The listing builds one solid part. Answer for the finished solid, in the listing's coordinates (mm). Face numbers are marked on the shaded views. A direction names the side the tool comes from. Give positions to 0.01 mm unless a question says otherwise; leave off trailing zeros. Write each loop counter-clockwise with the first axis right and the second up, starting at its lowest first coordinate (ties: lowest second). Pieces come first, ordered by that corner, then holes. Notation, with made-up numbers: M 53.5,52 L 94.5,52 A15 cw 94.5,71 Z; hole C 16,74.25 d3. An arc over 180 degrees is marked long. Answer as a JSON object with one key per item and string values.
Autodesk Inventor part; units mm, degrees
ref_plane "YZ Plane" through (0, 0, 0) normal (1, 0, 0) x (0, 1, 0)
ref_plane "XZ Plane" through (0, 0, 0) normal (0, 1, 0) x (-1, 0, 0)
ref_plane "XY Plane" through (0, 0, 0) normal (0, 0, 1) x (1, 0, 0)
sketch "Esquisse1" plane through (0, 0, 0) normal (0, 1, 0) x (-1, 0, 0)
  line L0 (0, 5) -> (40, 5)
  line L1 (40, 5) -> (40, -5)
  line L2 (40, -5) -> (0, -5)
  line L3 (0, -5) -> (0, 5)
  line L4 (0, 5) -> (17.5, 5)
  line L5 (17.5, 5) -> (17.5, 19)
  line L6 (17.5, 19) -> (0, 19)
  line L7 (0, 19) -> (0, 5)
  line L8 (0, -5) -> (12.7, -5)
  line L9 (12.7, -5) -> (12.7, -12.2)
  line L10 (12.7, -12.2) -> (0, -12.2)
  line L11 (0, -12.2) -> (0, -5)
  line L12 (17.5, 5) -> (21.5, 5)
  line L13 (21.5, 5) -> (21.5, 7)
  line L14 (21.5, 7) -> (17.5, 7)
  line L15 (17.5, 7) -> (17.5, 5)
  line L16 (12.7, -5) -> (14.7, -5)
  line L17 (14.7, -5) -> (14.7, -7)
  line L18 (14.7, -7) -> (12.7, -7)
  line L19 (12.7, -7) -> (12.7, -5)
  line L20 (40, -5) -> (14.7, -5)
  line L21 (14.7, -5) -> (14.7, -7)
  line L22 (14.7, -7) -> (40, -7)
  line L23 (40, -7) -> (40, -5)
  line L24 (12.7, -12.2) -> (14.7, -12.2)
  line L25 (14.7, -12.2) -> (14.7, -7)
  line L26 (14.7, -7) -> (12.7, -7)
  line L27 (12.7, -7) -> (12.7, -12.2)
  line L28 (40, 5) -> (21.5, 5)
  line L29 (21.5, 5) -> (21.5, 7)
  line L30 (21.5, 7) -> (40, 7)
  line L31 (40, 7) -> (40, 5)
  line L32 (21.5, 7) -> (17.5, 7)
  line L33 (17.5, 7) -> (17.5, 19)
  line L34 (17.5, 19) -> (21.5, 19)
  line L35 (21.5, 19) -> (21.5, 7)
  line L36 (40, -5) -> (42, -5)
  line L37 (42, -5) -> (42, 5)
  line L38 (42, 5) -> (40, 5)
  line L39 (40, 5) -> (40, -5)
  line L40 (0, -12.2) -> (12.7, -12.2)
  line L41 (12.7, -12.2) -> (12.7, -12.7)
  line L42 (12.7, -12.7) -> (0, -12.7)
  line L43 (0, -12.7) -> (0, -12.2)
  line L44 (0, 19) -> (17.5, 19)
  line L45 (17.5, 19) -> (17.5, 19.5)
  line L46 (17.5, 19.5) -> (0, 19.5)
  line L47 (0, 19.5) -> (0, 19)
  line L48 (21.5, 19) -> (17.5, 19)
  line L49 (17.5, 19) -> (17.5, 19.5)
  line L50 (17.5, 19.5) -> (21.5, 19.5)
  line L51 (21.5, 19.5) -> (21.5, 19)
  line L52 (42, 5) -> (40, 5)
  line L53 (40, 5) -> (40, 7)
  line L54 (40, 7) -> (42, 7)
  line L55 (42, 7) -> (42, 5)
  line L56 (42, -5) -> (40, -5)
  line L57 (40, -5) -> (40, -7)
  line L58 (40, -7) -> (42, -7)
  line L59 (42, -7) -> (42, -5)
  line L60 (14.7, -12.2) -> (12.7, -12.2)
  line L61 (12.7, -12.2) -> (12.7, -12.7)
  line L62 (12.7, -12.7) -> (14.7, -12.7)
  line L63 (14.7, -12.7) -> (14.7, -12.2)
  line L64 (0, 19.5) -> (21.5, 19.5)
  line L65 (21.5, 19.5) -> (21.5, 25.5)
  line L66 (21.5, 25.5) -> (0, 25.5)
  line L67 (0, 25.5) -> (0, 19.5)
  line L68 (0, -12.7) -> (14.7, -12.7)
  line L69 (14.7, -12.7) -> (14.7, -18.7)
  line L70 (14.7, -18.7) -> (0, -18.7)
  line L71 (0, -18.7) -> (0, -12.7)
  line L72 (42, -7) -> (56, -7)
  line L73 (56, -7) -> (56, 7)
  line L74 (56, 7) -> (42, 7)
  line L75 (42, 7) -> (42, -7)
  arc A0 (56, 7) -> (21.5, 25.5) centre (10.75, -35.9662) ccw
  arc A1 (21.5, 25.5) -> (0, 25.5) centre (10.75, -35.9662) ccw construction
  arc A2 (0, -18.7) -> (14.7, -18.7) centre (7.35, 85.9876) ccw construction
  arc A3 (14.7, -18.7) -> (56, -7) centre (7.35, 85.9876) ccw
  point P0 (0, 0)
  point P1 (0, 0)
  dimension "d1" = 40
  dimension "d3" = 14
  dimension "d4" = 10
  dimension "d5" = 7.2
  dimension "d6" = 0.5
  dimension "d7" = 0.5
  dimension "d8" = 17.5
  dimension "d9" = 12.7
  dimension "d10" = 2
  dimension "d11" = 2
  dimension "d12" = 2
  dimension "d13" = 4
  dimension "d14" = 2
  dimension "d15" = 6
  dimension "d16" = 6
  dimension "d17" = 14
extrude "Extrusion1" add sketch "Esquisse1" along normal mid plane 26 contours L67 L66 L65 L50 L46 | L35 L51 L65 A0 L74 L54 L30 | L42 L62 L69 L70 L71 | L55 L74 L73 L72 L59 L37 | L22 L58 L72 A3 L69 L63 L25
mirror "Symétrie1" about plane through (0, 0, 0) normal (1, 0, 0) of "Extrusion1"
sketch "Esquisse4" plane through (-14.7, -13, -18.7) normal (0, 0, -1) x (-1, 0, 0)
  circle A0 centre (-14.7, 13) radius 9.5
  dimension "d25" = 19
extrude "Extrusion4" cut sketch "Esquisse4" against normal through all
sketch "Esquisse5" plane through (0, 13, 0) normal (0, 1, 0) x (1, 0, 0)
  circle A0 centre (19.7, 12) radius 3.5
  circle A1 centre (28.5, -14) radius 3.5
  line L0 (42, 7) -> (56, -7) construction
  line L1 (56, 7) -> (42, -7) construction
  circle A2 centre (49, 0) radius 3.5
  line L2 (21.5, -7) -> (35.5, -7) construction
  line L3 (35.5, -7) -> (35.5, -21) construction
  line L4 (35.5, -21) -> (21.5, -21) construction
  line L5 (21.5, -21) -> (21.5, -7) construction
  line L6 (14.7, 7) -> (24.7, 7) construction
  line L7 (24.7, 7) -> (24.7, 17) construction
  line L8 (24.7, 17) -> (14.7, 17) construction
  line L9 (14.7, 17) -> (14.7, 7) construction
  line L10 (14.7, 17) -> (24.7, 7) construction
  line L11 (24.7, 17) -> (14.7, 7) construction
  line L12 (21.5, -7) -> (35.5, -21) construction
  line L13 (35.5, -7) -> (21.5, -21) construction
  point P0 (0, 0)
  dimension "d28" = 7
  dimension "d29" = 7
  dimension "d36" = 7
  dimension "d37" = 10
  dimension "d38" = 10
  dimension "d39" = 14
  dimension "d40" = 14
  dimension "d41" = 14
  dimension "d60" = 28.5
extrude "Extrusion5" cut sketch "Esquisse5" against normal through all
mirror "Symétrie3" about plane through (0, 0, 0) normal (1, 0, 0) of "Extrusion5"
sketch "Esquisse7" plane through (-21.5, -13, 25.5) normal (0, 0, 1) x (1, 0, 0)
  circle A0 centre (21.5, 13) radius 9.5
  circle A1 centre (21.5, 13) radius 8.5
  circle A2 centre (21.5, 13) radius 11.5
  dimension "d44" = 1
  dimension "d45" = 2
extrude "Extrusion7" add sketch "Esquisse7" along normal blind 1 contours A0 | A2
chamfer "Chanfrein1" distance 1 angle 45 1 edges at (-11.5, 0, 26.5)
sketch "Esquisse8" plane through (-14.7, -13, -18.7) normal (0, 0, -1) x (-1, 0, 0)
  circle A0 centre (-14.7, 13) radius 9.5
  circle A1 centre (-14.7, 13) radius 11.5
  circle A2 centre (-14.7, 13) radius 8.5
  dimension "d51" = 1
  dimension "d52" = 2
extrude "Extrusion8" add sketch "Esquisse8" along normal blind 1 contours A0 | A1
chamfer "Chanfrein2" distance 1 angle 45 1 edges at (11.5, 0, -19.7)
sketch "Esquisse9" plane through (0, 0, 26.5) normal (0, 0, 1) x (1, 0, 0)
  circle A0 centre (0, 0) radius 8.5
  line L0 (-56, 13) -> (56, 13)
  line L1 (56, 13) -> (56, 0)
  line L2 (56, 0) -> (-56, 0)
  line L3 (-56, 0) -> (-56, 13)
  line L4 (-56, -13) -> (-56, 13)
  line L5 (56, -13) -> (56, 13)
  line L6 (-21.5, 13) -> (21.5, 13)
extrude "Extrusion9" cut sketch "Esquisse9" against normal through all contours L2 A0 | A0 L2 L3 L0 L1 picked at (2.1208, 1.8788)
properties part number "wheel_base"
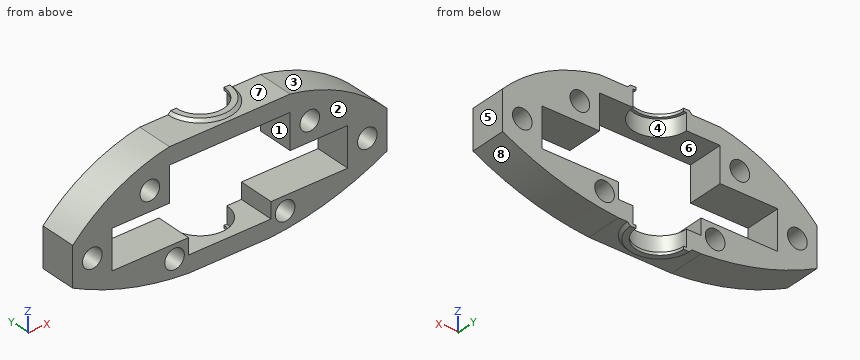
1. A cutting plane is placed at D-D, the plane x = -19.7. Give the vertices of the cut face in (y, z), plus the area to 3 significant figures.
Verdict:
{"outline": "M -13,-18.23 L 0,-18.23 L 0,-15.5 L -13,-15.5 Z; M -13,-8.5 L 0,-8.5 L 0,-7 L -13,-7 Z; M -13,19.5 L 0,19.5 L 0,25.5 L -13,25.5 Z", "area": "133 mm2"}
2. Consider line 1 along X through (y, z) = (-4.75, -5); line 2 along X through (y, z) = (-1.5, -9); line 3 along X through (y, z) = (-11, 14.5). Determine where each line is inside the solid, lowest interval first.
Verdict:
{"line 1": "x = -56 to -42, 42 to 56", "line 2": "x = -51.97 to -21.5, -17.9 to -14.7, 14.7 to 17.9, 21.5 to 51.97", "line 3": "x = -47.45 to -31.96, -25.04 to -21.5, 21.5 to 25.04, 31.96 to 47.45"}
3. A cutting plane is placed at B-B, the plane x = -37. Give the vertices of the cut face in (y, z), plus the area to 3 significant figures.
Verdict:
{"outline": "M -13,-14.68 L 0,-14.68 L 0,-7 L -13,-7 Z; M -13,7 L 0,7 L 0,20.64 L -13,20.64 Z", "area": "277 mm2"}
4. Flat-ended cylindrical pins translate along their axes: pin 1 (4 mm diameter, centred on x = -35.5, y = -9, fed in from -Z); pin 2 (4 mm diameter, centred on x = 34.5, y = -5, fed in from -Z); pin 3 (3 mm diameter, centred on y = -8, z = 17, fed in from +X). Find the tip coordinate at first contact, or state that the pin passes through.
Verdict:
{"pin 1": "stops at z = -15.65", "pin 2": "stops at z = -15.9", "pin 3": "stops at x = 46.03"}
5. The mould has two halves that part along Z. Classify the marked faces 1, 2 and 3: released by +Z, released by -Z, zero draft, split by the parting line, or undercut.
Verdict:
{"face 1": "undercut", "face 2": "zero draft", "face 3": "released by +Z"}
6. For the marked faces 4, 5, 6, 7 and 8, determine the directions among +Z, -Z, +X, -X, +Y, -Y from which every point of the face is accessible in a straight line to the end or side of a thin tool.
Verdict:
{"face 4": "+Y", "face 5": "+Z, -Z, +X, +Y, -Y", "face 6": "+Y, -Y", "face 7": "+Z, -Y", "face 8": "-Z, +X, +Y, -Y"}
7. A cutting plane is placed at A-A, the plane z = 0. Give the vertices of the cut face in (x, y).
Verdict:
{"outline": "M -56,-13 L -52.5,-13 L -52.5,0 L -56,0 Z; M -45.5,-13 L -42,-13 L -42,0 L -45.5,0 Z; M 42,-13 L 45.5,-13 L 45.5,0 L 42,0 Z; M 52.5,-13 L 56,-13 L 56,0 L 52.5,0 Z"}
8. A cutting plane is placed at C-C, the plane y = -6.25. Count the separate pieces of the cut face and the enclosed holes in it, plus the area to 3 significant figures.
Verdict:
{"separate pieces": "2", "enclosed holes": "6", "area": "1,850 mm2"}
